from build123d import *

# Parameters (mm, degrees)
F0_W     = 8
F0_H     = 25
F1_DEPTH = 2
F2_W     = 3.3
F2_H     = 18.2
F3_DEPTH = 0.5
F5_DEPTH = 8.001
F6_R     = 1


with BuildPart() as f1:
    # F0 (on Top) → F1 (new body)
    with BuildSketch(Plane.XY):
        with Locations((-4, 12.5)):
            Rectangle(F0_W, F0_H)
    extrude(amount=F1_DEPTH)

    # F2 (on face) → F3 (cut)
    with BuildSketch(Plane(origin=(0, 0, 0), x_dir=(1, 0, 0), z_dir=(0, 0, -1))):
        Polygon((-7.1, -6.8), (-5.8275572956, -6.8), (-2.5275572956, -6.8), (-0.9, -6.8), (-0.9, 0), (-7.1, 0), align=None)
        with Locations((-4.1775572956, -15.9)):
            Rectangle(F2_W, F2_H)
    extrude(amount=-F3_DEPTH, mode=Mode.SUBTRACT)

    # F4 (on face) → F5 (cut, through all)
    with BuildSketch(Plane.YZ):
        Polygon((6.8, 0), (0, 0.5), (0, 0), align=None)
    extrude(amount=-F5_DEPTH, mode=Mode.SUBTRACT)

    # F6
    f6_edges = [f1.edges().sort_by_distance(p)[0] for p in [
        (0, 25, 1),
        (-8, 25, 1),
        (-4, 25, 2),
        (0, 12.5, 2),
        (-8, 12.5, 2),
        (-4, 0, 2),
    ]]
    fillet(f6_edges, radius=F6_R)


solid = f1.part
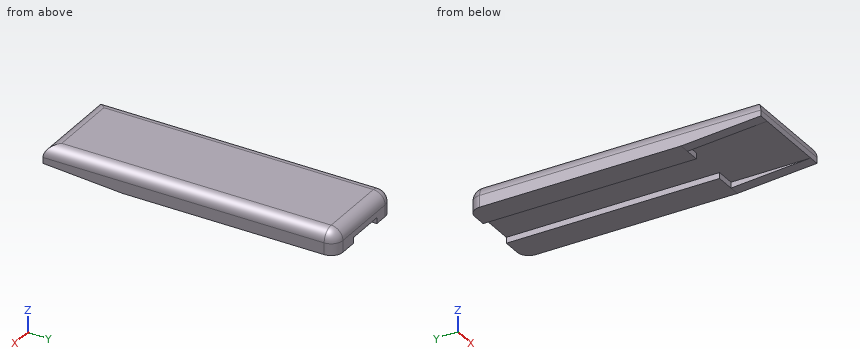
Can you work these out from the model? Positions are in its coordinate system, mm. Coordinates: 2 decimals unless noted, no trailing zeros. Loops run counter-clockwise (first coordinate to the right, second up) from the corner with the lowest first, then second, coordinate; pieces in that order, holes last. Notation, with made-up numbers: (47, 63.5) - (88, 63.5) arc R18 cw to (88, 72.5) - close; hole circle Ø9 at (65, -2.75). An arc over 180 degrees is marked (long way). Put each result on its own line as item: value. Start each with the question number.
Item 1: Suppose I cut it at B-B (y = 14). Please give me the cut outline in (x, z), and give its area (3 significant figures).
Item 2: Suppose I cut it at A-A (x = -1.25). Please give me the cut outline in (y, z).
Item 3: Suppose I cut it at D-D (x = -4.5). Please give me the cut outline in (y, z), and give its area (3 significant figures).
Item 4: Suppose I cut it at C-C (z = 1.4). Please give me the cut outline in (x, y).
Item 5: If I drill on line 1 along Z through (x, y) = (-5.5, 15); line 2 along Y through (x, z) = (-2.5, 1.05); line 3 along Y through (x, z) = (-7, 0.3), over which ranges is the centre line in solid material (lowest first)?
Here are the results:
1. outline: (-8, 0) - (-5.83, 0) - (-5.83, 0.5) - (-2.53, 0.5) - (-2.53, 0) - (0, 0) - (0, 1) arc R1 ccw to (-1, 2) - (-7, 2) arc R1 ccw to (-8, 1) - close
1. area: 13.9 mm²
2. outline: (0, 0.5) - (6.8, 0.5) - (6.8, 0) - (25, 0) - (25, 1) arc R1 ccw to (24, 2) - (1, 2) arc R1 ccw to (0, 1) - close
3. outline: (0, 0.5) - (25, 0.5) - (25, 1) arc R1 ccw to (24, 2) - (1, 2) arc R1 ccw to (0, 1) - close
3. area: 37.1 mm²
4. outline: (-7.92, 0.08) - (-0.08, 0.08) - (-0.08, 24) arc R0.92 ccw to (-1, 24.92) - (-7, 24.92) arc R0.92 ccw to (-7.92, 24) - close
5. line 1: 0.5 to 2
5. line 2: 0 to 25
5. line 3: 6.8 to 25
